Build history of the part. All positions in model axes, mm. Give positions to 0.01 mm unless a question says otherwise; leave off trailing zeros. Loops run counter-clockwise (first coordinate to the right, second up) from the corner with the lowest first, then second, coordinate; pieces in that order, holes last. Notation, with made-up numbers: (37.25, 81) -> (77.25, 81) arc R12 ccw to (77.25, 98) -> close; hole circle Ø6 at (15.25, 20). An arc over 180 degrees is marked (long way). Answer as a JSON object with one key per item and string values. Group by question number.
Q1. Band-saw the part on B-B, the plane y = 7.62. Write the cut outline in (x, z) (3 decimals).
Q2. Two-plate mould, pull along Y, no slides. Class faces 1 (the cylindrical face through (1.565, 7.511, -5.133)), 2 (the flat face through (2, 0, -26)), 3 (the flat face through (0, 44, -25)): pulls with the +Y half, pulls with the -Y half, needs draft (parallel to the pull), parting line crosses it, or undercut.
Q3. Band-saw the part on C-C, the plane x = 1.9. Write the cut outline in (y, z).
Q4. Wall check: probe 1 along Z at (x, y) = (2.1, 7.62); probe 2 along Y at (x, z) = (1.55, -7.62); probe 3 along Z at (x, y) = (0.5, 81.5). Give the ranges that are in metal, low to high. Write a range as from..to.
Q5. Drop flat-ended pins along their axis: pin 1 (8 mm diameter, centred on y = 82.25, z = -7.62, fed in from -X); pin 2 (3 mm diameter, centred on y = 82.25, z = -43.18, fed in from -X). Give the stop position or say it passes through.
Q6. Band-saw the part on A-A, the plane z = -7.62. Write the cut outline in (x, y) (3 decimals).
Autodesk Inventor part; units mm, degrees
ref_plane "YZ Plane" through (0, 0, 0) normal (1, 0, 0) x (0, 1, 0)
ref_plane "XZ Plane" through (0, 0, 0) normal (0, 1, 0) x (-1, 0, 0)
ref_plane "XY Plane" through (0, 0, 0) normal (0, 0, 1) x (1, 0, 0)
sketch "Sketch1" plane through (0, 0, 0) normal (1, 0, 0) x (0, 1, 0)
  line L0 (0, 0) -> (89.8652, 0)
  line L1 (89.8652, 0) -> (89.8652, -50.8)
  line L2 (89.8652, -50.8) -> (0, -50.8)
  line L3 (0, -50.8) -> (0, 0)
  dimension "d0" = 89.8652
  dimension "d1" = 50.8
extrude "Extrusion1" add sketch "Sketch1" along normal blind 3.175
sketch "Sketch2" plane through (3.175, 0, 0) normal (1, 0, 0) x (0, 0, -1)
  line L0 (0, 89.8652) -> (0, 0)
  line L1 (50.8, 89.8652) -> (0, 89.8652)
  point P0 (7.62, 82.2452)
  dimension "d4" = 7.62
  dimension "d5" = 7.62
hole "Hole1" at (3.175, 82.2452, -7.62) direction (-1, 0, 0) diameter 4.9784 end through all
pattern_linear "Rectangular Pattern1" count 2 spacing 74.6252 along (0, -1, 0) count 2 spacing 35.56 along (0, 0, -1) of "Hole1"
properties part number "arm to water block plate" material "Aluminum 6061"
Worked answers:
{
 "1": {"outline": "(0, -50.8) -> (3.175, -50.8) -> (3.175, -45.669) -> (0, -45.669) -> close; (0, -40.691) -> (3.175, -40.691) -> (3.175, -10.109) -> (0, -10.109) -> close; (0, -5.131) -> (3.175, -5.131) -> (3.175, 0) -> (0, 0) -> close"},
 "2": {"face 1": "undercut", "face 2": "pulls with the -Y half", "face 3": "needs draft"},
 "3": {"outline": "(0, -50.8) -> (89.87, -50.8) -> (89.87, 0) -> (0, 0) -> close; hole circle Ø4.98 at (7.62, -43.18); hole circle Ø4.98 at (7.62, -7.62); hole circle Ø4.98 at (82.25, -43.18); hole circle Ø4.98 at (82.25, -7.62)"},
 "4": {"probe 1": "-50.8..-45.67, -40.69..-10.11, -5.13..0", "probe 2": "0..5.13, 10.11..79.76, 84.73..89.87", "probe 3": "-50.8..-45.56, -40.8..-10, -5.24..0"},
 "5": {"pin 1": "x = 0", "pin 2": "through"},
 "6": {"outline": "(0, 0) -> (3.175, 0) -> (3.175, 5.131) -> (0, 5.131) -> close; (0, 10.109) -> (3.175, 10.109) -> (3.175, 79.756) -> (0, 79.756) -> close; (0, 84.734) -> (3.175, 84.734) -> (3.175, 89.865) -> (0, 89.865) -> close"}
}
